Geometry: final body of the model. Coordinates: model frame, mm. Give positions to 0.01 mm unless a question says otherwise; leave off trailing zeros. Write each loop counter-clockwise with the first axis right and the second up, starting at its lowest first coordinate (ties: lowest second). Pieces come first, ordered by that corner, then holes.
Autodesk Inventor part; units mm, degrees
ref_plane "YZ Plane" through (0, 0, 0) normal (1, 0, 0) x (0, 1, 0)
ref_plane "XZ Plane" through (0, 0, 0) normal (0, 1, 0) x (-1, 0, 0)
ref_plane "XY Plane" through (0, 0, 0) normal (0, 0, 1) x (1, 0, 0)
sketch "Sketch1" plane through (0, 0, 0) normal (0, 0, 1) x (1, 0, 0)
  line L0 (-65, -65) -> (65, -65)
  line L1 (65, -65) -> (65, 65)
  line L2 (65, 65) -> (-65, 65)
  line L3 (-65, 65) -> (-65, -65)
  line L4 (-65, -65) -> (65, 65) construction
  line L5 (65, -65) -> (-65, 65) construction
  point P0 (0, 0)
  dimension "d0" = 130
  dimension "d1" = 130
extrude "Extrusion1" add sketch "Sketch1" along normal blind 12
sketch "Sketch2" plane through (0, 0, 12) normal (0, 0, 1) x (1, 0, 0)
  line L0 (-65, -65) -> (65, -65)
  line L1 (65, -65) -> (65, 65)
  line L2 (65, 65) -> (-65, 65)
  point P0 (0, 0)
  point P1 (40, -40)
  point P2 (40, 40)
  point P3 (0, 40)
  point P4 (-40, 40)
  point P5 (-40, -40)
  point P6 (0, -40)
  dimension "d4" = 40
  dimension "d5" = 40
  dimension "d7" = 25
  dimension "d8" = 25
  dimension "d9" = 25
hole "Hole1" at (40, -40, 12) at (40, 40, 12) at (0, 40, 12) at (-40, 40, 12) at (-40, -40, 12) at (0, -40, 12) direction (0, 0, -1) diameter 4.917 end through all
sketch "Sketch3" plane through (0, 0, 12) normal (0, 0, 1) x (1, 0, 0)
  line L0 (-1.5, 20) -> (23.5, 20)
  line L1 (23.5, 20) -> (23.5, -20)
  line L2 (23.5, -20) -> (-1.5, -20)
  line L3 (-1.5, -20) -> (-1.5, 20)
  line L4 (65, -65) -> (65, 65)
  point P0 (0, 0)
  point P1 (-1.5, 0)
  dimension "d17" = 40
  dimension "d18" = 25
  dimension "d19" = 41.5
hole "Hole2" at (23.5, 20, 12) at (-1.5, 20, 12) at (-1.5, -20, 12) at (23.5, -20, 12) direction (0, 0, -1) diameter 4.5 end through all
sketch "Sketch4" plane through (0, 0, 12) normal (0, 0, 1) x (1, 0, 0)
  line L0 (-20, 40) -> (20, 40)
  line L1 (20, 40) -> (20, -40)
  line L2 (20, -40) -> (-20, -40)
  line L3 (-20, -40) -> (-20, 40)
  circle A0 centre (40, -40) radius 2.4585
  circle A1 centre (0, -40) radius 2.4585
  circle A2 centre (0, 40) radius 2.4585
  point P0 (0, 0)
  dimension "d27" = 40
  dimension "d28" = 20
hole "Hole3" at (20, -40, 12) at (-20, -40, 12) at (-20, 40, 12) at (20, 40, 12) direction (0, 0, -1) diameter 4.917 end through all
sketch "Sketch5" plane through (0, 0, 0) normal (0, 0, -1) x (-1, 0, 0)
  line L0 (40, -50) -> (-40, -50)
  line L1 (-40, -50) -> (-40, 50)
  line L2 (-40, 50) -> (40, 50)
  line L3 (40, 50) -> (40, -50)
  line L4 (-65, -65) -> (-65, 65)
  line L5 (-65, 65) -> (65, 65)
  line L6 (65, -65) -> (-65, -65)
  line L7 (65, 65) -> (65, -65)
  point P0 (0, 0)
  dimension "d36" = 25
  dimension "d38" = 15
  dimension "d39" = 15
  dimension "d40" = 25
hole "Hole4" at (-40, -50, 0) at (40, -50, 0) at (40, 50, 0) at (-40, 50, 0) direction (0, 0, 1) diameter 4.134 end through all
equation "\"d28\" = 0.5 * d27"
equation "\"d39\" = d38"
equation "\"d40\" = d36"
properties part number "Befestigungsplatte" material "Aluminum 6061"
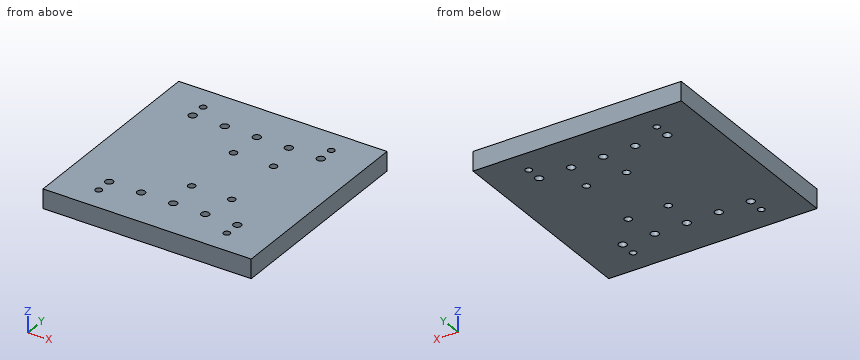
Q1. Section A-A on y = -40. Output: boundary loops of the cut face in (x, z), plus the area to 3 significant figures.
Filled sheet:
outline: (-65, 0) - (-42.46, 0) - (-42.46, 12) - (-65, 12) - close; (-37.54, 0) - (-22.46, 0) - (-22.46, 12) - (-37.54, 12) - close; (-17.54, 0) - (-2.46, 0) - (-2.46, 12) - (-17.54, 12) - close; (2.46, 0) - (17.54, 0) - (17.54, 12) - (2.46, 12) - close; (22.46, 0) - (37.54, 0) - (37.54, 12) - (22.46, 12) - close; (42.46, 0) - (65, 0) - (65, 12) - (42.46, 12) - close
area: 1,260 mm2
Q2. Section C-C on z = 9.75. Count the separate pieces of the cut face and the enclosed holes in it, plus the area to 3 significant figures.
Filled sheet:
separate pieces: 1
enclosed holes: 18
area: 16,600 mm2
Q3. Section B-B on x = 40. Output: boundary loops of the cut face in (y, z).
Filled sheet:
outline: (-65, 0) - (-52.07, 0) - (-52.07, 12) - (-65, 12) - close; (-47.93, 0) - (-42.46, 0) - (-42.46, 12) - (-47.93, 12) - close; (-37.54, 0) - (37.54, 0) - (37.54, 12) - (-37.54, 12) - close; (42.46, 0) - (47.93, 0) - (47.93, 12) - (42.46, 12) - close; (52.07, 0) - (65, 0) - (65, 12) - (52.07, 12) - close
Q4. Ray query, line 1 along X through (y, z) = (-40, 8.75); line 2 along X through (y, z) = (50, 3.25); line 3 along Y through (x, z) = (40, 3.5). Return the intervals inside material, ascending.
Filled sheet:
line 1: x = -65 to -42.46, -37.54 to -22.46, -17.54 to -2.46, 2.46 to 17.54, 22.46 to 37.54, 42.46 to 65
line 2: x = -65 to -42.07, -37.93 to 37.93, 42.07 to 65
line 3: y = -65 to -52.07, -47.93 to -42.46, -37.54 to 37.54, 42.46 to 47.93, 52.07 to 65
Q5. Section D-D on y = 20. Output: boundary loops of the cut face in (x, z).
Filled sheet:
outline: (-65, 0) - (-3.75, 0) - (-3.75, 12) - (-65, 12) - close; (0.75, 0) - (21.25, 0) - (21.25, 12) - (0.75, 12) - close; (25.75, 0) - (65, 0) - (65, 12) - (25.75, 12) - close
Q6. Pin query (flat end, axial travel): P1, Ø4.5, axis at x = 20, y = 40, coming from the +Z side; P2, Ø6.5, axis at x = -40, y = -40, coming from the +Z side. Return the tip coordinate at first contact, or that it passes through.
Filled sheet:
P1: passes through
P2: stops at z = 12
